Check sheet for the modelled part. Datum: model origin and axes. Units: mm. Round coordinates to 2 decimals unless told otherwise and drop trailing zeros. Write each loop counter-clockwise with the first axis right and the second up, starting at its lowest first coordinate (ties: lowest second). Pieces come first, ordered by that corner, then holes. Notation, with made-up numbers: (59.5, -18.5) -> (84.5, -18.5) arc R22 ccw to (84.5, 5.5) -> close; hole circle Ø6 at (20.25, 80). An arc over 180 degrees is marked (long way). Answer as a JSON object with one key per item and string values. Group by question number.
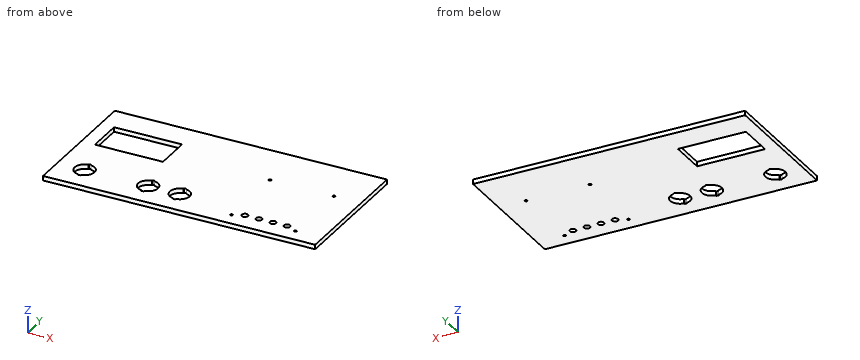
```python
from build123d import *

# Parameters (mm, degrees)
SKIZZE1_W                       = 300
SKIZZE1_H                       = 150
AUFSATZ_LINEAR_AUSTRAGEN1_DEPTH = 5
SKIZZE3_W                       = 75
SKIZZE3_H                       = 40
SCHNITT_LINEAR_AUSTRAGEN2_DEPTH = 168.779617356
SKIZZE5_R                       = 11
SKIZZE5_W                       = 3
SKIZZE5_H                       = 24
SCHNITT_LINEAR_AUSTRAGEN4_DEPTH = 168.779617356
SKIZZE2_R                       = 1.375
SKIZZE2_R_2                     = 3.35
SCHNITT_LINEAR_AUSTRAGEN5_DEPTH = 168.779617356


with BuildPart() as part:
    # Skizze1 → Aufsatz-Linear austragen1 (new body)
    with BuildSketch(Plane.XY):
        Rectangle(SKIZZE1_W, SKIZZE1_H)
    extrude(amount=AUFSATZ_LINEAR_AUSTRAGEN1_DEPTH)

    # Skizze3 → Schnitt-Linear austragen2 (cut, through all)
    with BuildSketch(Plane.XY.offset(5)):
        with Locations((-97.5, 25)):
            Rectangle(SKIZZE3_W, SKIZZE3_H)
    extrude(amount=-SCHNITT_LINEAR_AUSTRAGEN2_DEPTH, mode=Mode.SUBTRACT)

    # Skizze5 → Schnitt-Linear austragen4 (cut, through all)
    with BuildSketch(Plane.XY.offset(5)):
        with Locations((-15, -45)):
            Circle(SKIZZE5_R)
        with Locations((-50, -45)):
            Circle(SKIZZE5_R)
        with Locations((-120, -45)):
            Circle(SKIZZE5_R)
        with Locations((-15, -45)):
            Rectangle(SKIZZE5_W, SKIZZE5_H)
        with Locations((-50, -45)):
            Rectangle(SKIZZE5_W, SKIZZE5_H)
        with Locations((-120, -45)):
            Rectangle(SKIZZE5_W, SKIZZE5_H)
    extrude(amount=-SCHNITT_LINEAR_AUSTRAGEN4_DEPTH, mode=Mode.SUBTRACT)

    # Skizze2 → Schnitt-Linear austragen5 (cut, through all)
    with BuildSketch(Plane.XY.offset(5)):
        with Locations((49.537329599, 20.961824544)):
            Circle(SKIZZE2_R)
        with Locations((119.962670401, 20.961824544)):
            Circle(SKIZZE2_R)
        with Locations((119.962670401, -59.261824544)):
            Circle(SKIZZE2_R)
        with Locations((49.537329599, -59.261824544)):
            Circle(SKIZZE2_R)
        with Locations((61.5, -54)):
            Circle(SKIZZE2_R_2)
        with Locations((77, -54)):
            Circle(SKIZZE2_R_2)
        with Locations((92.5, -54)):
            Circle(SKIZZE2_R_2)
        with Locations((108, -54)):
            Circle(SKIZZE2_R_2)
    extrude(amount=-SCHNITT_LINEAR_AUSTRAGEN5_DEPTH, mode=Mode.SUBTRACT)


solid = part.part
```
(1) Section check D-D on z = 1.85. State how many separate pieces and enclosed holes the cut face has, then the cut area to 3 significant figures.
(2) Section check B-B on x = -91.5. Record the cut outline in (y, z), then the cut area to 3 significant figures.
(3) Go/stop test with a flat-tipped pin: pin 1 Ø4 at (x, y) = (61.5, -54) entering from -Z. Record where the tip stops, or that it passes through.
(4) Section check A-A on y = 41.5. Record the cut outline in (x, z), then the cut area to 4 significant figures.
(5) Section check C-C on y = -42. Record the cut outline in (x, z).
(6) Scan lines: line 1 along Y through (x, z) = (92.5, 1.9); line 2 along X through (y, z) = (9, 1); line 3 along Y through (x, z) = (-70, 4.6). Record each from-to range of solid material in increasing order.
Data:
{
 "1": {"separate pieces": "1", "enclosed holes": "12", "area": "40,700 mm²"},
 "2": {"outline": "(-75, 0) -> (5, 0) -> (5, 5) -> (-75, 5) -> close; (45, 0) -> (75, 0) -> (75, 5) -> (45, 5) -> close", "area": "550 mm²"},
 "3": {"pin 1": "passes through"},
 "4": {"outline": "(-150, 0) -> (-135, 0) -> (-135, 5) -> (-150, 5) -> close; (-60, 0) -> (150, 0) -> (150, 5) -> (-60, 5) -> close", "area": "1,125 mm²"},
 "5": {"outline": "(-150, 0) -> (-130.58, 0) -> (-130.58, 5) -> (-150, 5) -> close; (-109.42, 0) -> (-60.58, 0) -> (-60.58, 5) -> (-109.42, 5) -> close; (-39.42, 0) -> (-25.58, 0) -> (-25.58, 5) -> (-39.42, 5) -> close; (-4.42, 0) -> (150, 0) -> (150, 5) -> (-4.42, 5) -> close"},
 "6": {"line 1": "y = -75 to -57.35, -50.65 to 75", "line 2": "x = -150 to -135, -60 to 150", "line 3": "y = -75 to 5, 45 to 75"}
}
